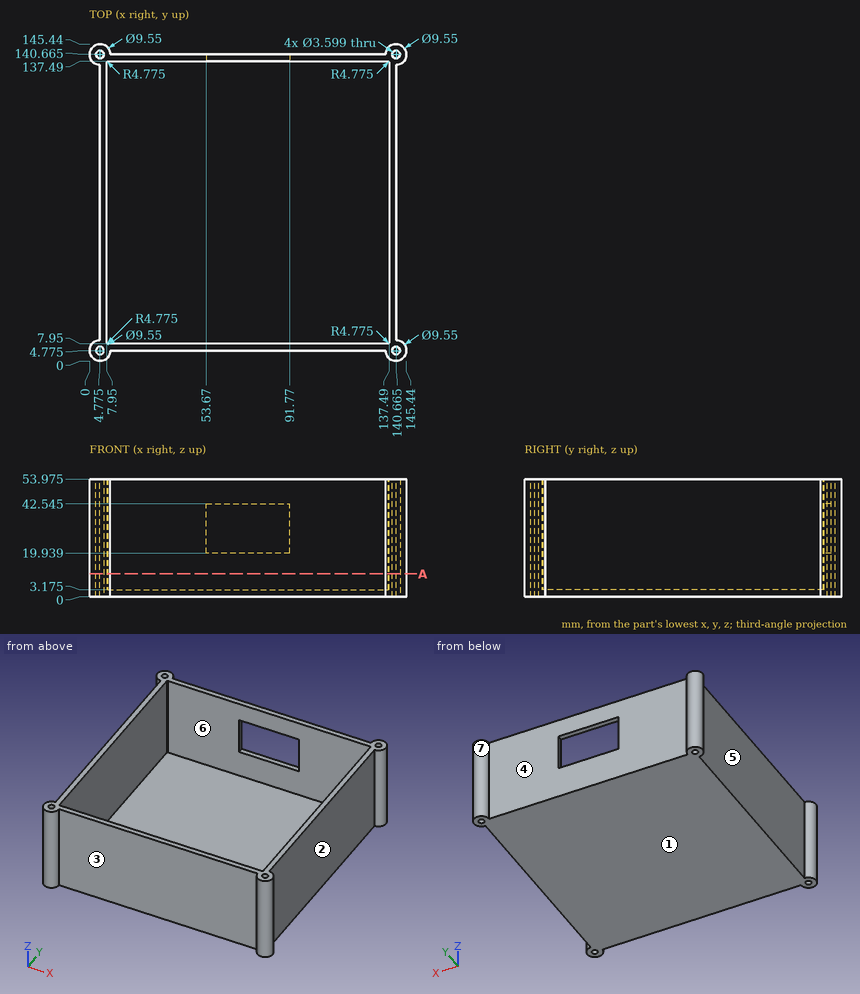
Check sheet for the drawn part. Datum: minimum x, y, z corner. Units: mm. A direction names the side the tool comes from. Round coordinates to 2 decimals unless told otherwise and drop trailing zeros.
(1) Scan lines: probe 1 along Z at (x, y) = (73, 140) (1 decimal); probe 2 along Z at (x, y) = (107, 75.5) (1 decimal); probe 3 along Y at (x, z) = (8, 17) (1 decimal). Record each from-to range of solid material in increasing order.
(2) Access from +Z, -Z, +X, -X, +Y, -Y to the whole of each face (thin tool, end or side, straight path). Record for the marked faces 5, 6 and 7.
(3) Go/stop test with flat-tipped pins: P1, Ø16, axis at x = 43, z = 16.5, coming from the -Y side (1 decimal); P2, Ø3, axis at x = 140.67, y = 140.67, coming from the +Z side; P3, Ø1.6, axis at y = 138.5, z = 26, coming from the -X side; P4, Ø2.5, axis at y = 139.5, z = 35.5, coming from the +X side. Record where each tip stops, or that it passes through.
(4) Draft check along Y on the marked faces 1, 2, 3 and 4. Enter one of: pulls with the +Y half, pulls with the -Y half, needs draft (parallel to the pull), parting line crosses it, or undercut.
(5) Cross-section at A-A, the plane z = 10.5. State how many separate pieces and enclosed holes the cut face has, and give its area (3 significant figures).
Check sheet entries:
1. probe 1: z = 0 to 19.9, 42.5 to 54
1. probe 2: z = 0 to 3.2
1. probe 3: y = 1.3 to 8.3, 137.1 to 144.2
2. face 5: +Z, -Z, -X
2. face 6: +Z
2. face 7: +Z, -Z
3. P1: stops at y = 4.8
3. P2: passes through
3. P3: stops at x = 0.2
3. P4: stops at x = 145.44
4. face 1: needs draft
4. face 2: undercut
4. face 3: pulls with the -Y half
4. face 4: pulls with the +Y half
5. separate pieces: 1
5. enclosed holes: 5
5. area: 1,860 mm2
